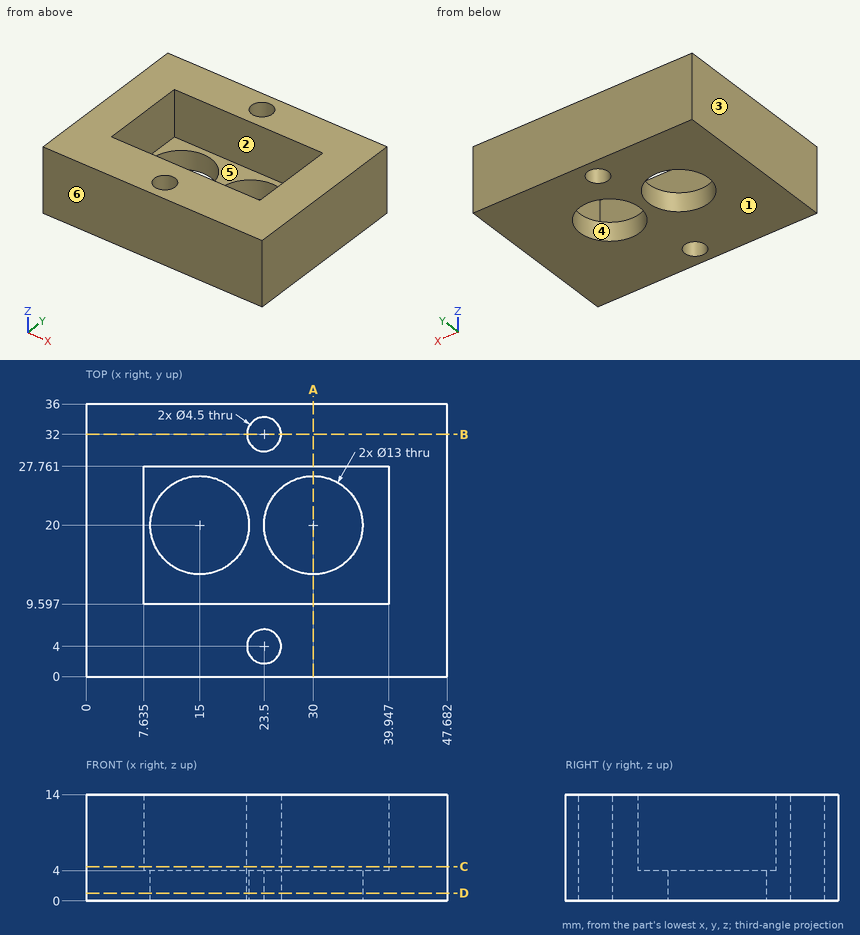
Geometry: see drawing. Coordinates: mm, zero at the bounding-box minimum. A direction names the side the tool comes from. Give positions to 0.01 mm unless a question says otherwise; leave off trailing zeros. Write each loop counter-clockwise with the first axis right and the second up, starting at its lowest first coordinate (ties: lowest second). Pieces come first, ordered by that corner, then holes. Notation, with made-up numbers: M -17,30.5 L 13,30.5 A32 ccw 13,57.5 Z; hole C 25.5,-15.75 d3. An arc over 180 degrees is marked long. Return JSON: item names as keys, results as strings. Group by question number.
1) Cut plane A-A, the plane x = 30. Output: boundary loops of the cut face in (y, z).
2) Draft query along X for the marked faces 3, 4, 5 and 6. Return one class per face: released by +X, released by -X, zero draft, split by the parting line, or undercut.
3) Ray query, L1, parallel to Y at x = 23.5, z = 10.5; L2, parallel to X at y = 19, z = 9.75 (1 decimal); L3, parallel to Y at x = 15, z = 1.6. Return the intervals inside material, ascending.
4) Cut plane C-C, the plane z = 4.5. Give the number of separate pieces and of enclosed holes in the cut face, then the cut area to 3 significant figures.
5) Cut plane B-B, the plane y = 32. Output: boundary loops of the cut face in (x, z).
6) Set-up query: the marked faces 1 and 2. Return all of +Z, -Z, +X, -X, +Y, -Y with unobstructed straight access to the full face (end or side cutting, diameter ignored); none if empty.
7) Cut plane D-D, the plane z = 1. Output: boundary loops of the cut face in (x, y).
8) First-contact query: pin 1 Ø11.5 at (x, y) = (30, 20) entering from -Z. Flat tip, straight axial feed; report the tip coordinate or a pass-through.
Data:
{
 "1": {"outline": "M 0,0 L 13.5,0 L 13.5,4 L 9.6,4 L 9.6,14 L 0,14 Z; M 26.5,0 L 36,0 L 36,14 L 27.76,14 L 27.76,4 L 26.5,4 Z"},
 "2": {"face 3": "released by -X", "face 4": "undercut", "face 5": "undercut", "face 6": "zero draft"},
 "3": {"L1": "y = 0 to 1.75, 6.25 to 9.6, 27.76 to 29.75, 34.25 to 36", "L2": "x = 0 to 7.6, 39.9 to 47.7", "L3": "y = 0 to 13.5, 26.5 to 36"},
 "4": {"separate pieces": "1", "enclosed holes": "3", "area": "1,100 mm²"},
 "5": {"outline": "M 0,0 L 21.25,0 L 21.25,14 L 0,14 Z; M 25.75,0 L 47.68,0 L 47.68,14 L 25.75,14 Z"},
 "6": {"face 1": "-Z, +X, -X, +Y, -Y", "face 2": "+Z"},
 "7": {"outline": "M 0,0 L 47.68,0 L 47.68,36 L 0,36 Z; hole C 15,20 d13; hole C 23.5,4 d4.5; hole C 23.5,32 d4.5; hole C 30,20 d13"},
 "8": {"pin 1": "passes through"}
}
